Autodesk Inventor part; units mm, degrees
ref_plane "YZ Plane" through (0, 0, 0) normal (1, 0, 0) x (0, 1, 0)
ref_plane "XZ Plane" through (0, 0, 0) normal (0, 1, 0) x (-1, 0, 0)
ref_plane "XY Plane" through (0, 0, 0) normal (0, 0, 1) x (1, 0, 0)
sketch "Skizze1" plane through (0, 0, 0) normal (0, 0, 1) x (1, 0, 0)
  line L0 (-126, 0) -> (126, 0)
  line L1 (0, -126) -> (0, 126)
  line L2 (-90, 4.7809) -> (90, 4.7809)
  line L3 (90, 4.7809) -> (90, -5.2191)
  line L4 (90, -5.2191) -> (-90, -5.2191)
  line L5 (-90, -5.2191) -> (-90, 4.7809)
  line L6 (-4.0898, 90) -> (5.9102, 90)
  line L7 (5.9102, 90) -> (5.9102, -90)
  line L8 (5.9102, -90) -> (-4.0898, -90)
  line L9 (-4.0898, -90) -> (-4.0898, 90)
  point P0 (0, 0)
  point P1 (-4.0898, 4.7809)
  point P2 (-4.0898, -5.2191)
  point P3 (5.9102, -5.2191)
  point P4 (5.9102, 4.7809)
  dimension "d0" = 10
  dimension "d1" = 180
  dimension "d2" = 90
  dimension "d3" = 10
  dimension "d4" = 180
  dimension "d5" = 90
extrude "Extrusion1" add sketch "Skizze1" along normal blind 190
sketch "Skizze2" plane through (0, 0, 0) normal (0, 0, -1) x (-1, 0, 0)
  line L0 (-90, 4.7809) -> (-5.9102, 4.7809)
  line L1 (90, -5.2191) -> (4.0898, -5.2191)
  line L2 (-5.9102, 4.7809) -> (4.0898, 4.7809)
  line L3 (4.0898, 4.7809) -> (4.0898, -5.2191)
  line L4 (4.0898, -5.2191) -> (-5.9102, -5.2191)
  line L5 (-5.9102, -5.2191) -> (-5.9102, 4.7809)
  point P0 (0, 0)
extrude "Extrusion2" add sketch "Skizze2" along normal blind 7
properties part number "Gitter"
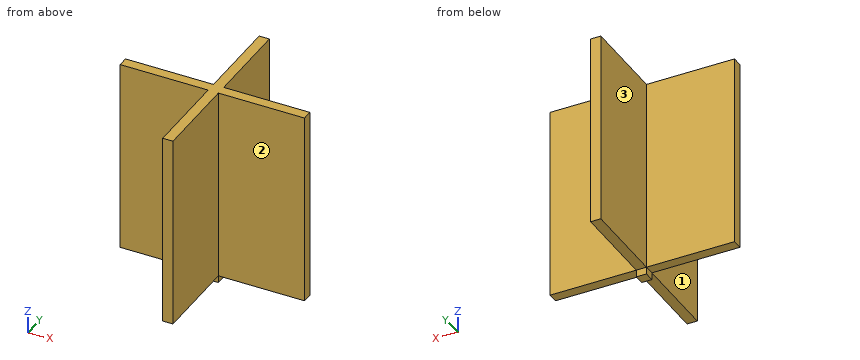
Check sheet for the modelled part. Datum: model origin and axes. Units: mm. Face numbers are marked on the shaded views. A direction names the side the tool comes from. Coordinates: 2 decimals unless noted, no trailing zeros. Write each loop counter-clockwise with the first axis right and the second up, starting at its lowest first coordinate (ties: lowest second). Pieces come first, ordered by that corner, then holes. Notation, with made-up numbers: (-30.75, -22.75) -> (-7.75, -22.75) arc R23 cw to (-7.75, -1.75) -> close; hole circle Ø8 at (54.25, 13.5). An arc over 180 degrees is marked (long way). Use a Markdown table: item, result.
1. Go/stop test with flat-tipped pins: pin 1 Ø10 at (x, z) = (-26, 20.5) entering from -Y; pin 2 Ø3.5 at (y, z) = (0.5, -2) entering from +X; pin 3 Ø3 at (x, y) = (1.5, 57) entering from -Z. Record where each tip stops, or that it passes through.
Reported:
| item | result |
|---|---|
| pin 1 | stops at y = -5.22 |
| pin 2 | stops at x = 5.91 |
| pin 3 | stops at z = 0 |
2. Sectioned sample at C-C (y = 53). Enter the section's corners in (x, z), plus the area to 3 significant figures.
Reported:
| item | result |
|---|---|
| outline | (-4.09, 0) -> (5.91, 0) -> (5.91, 190) -> (-4.09, 190) -> close |
| area | 1,900 mm2 |
3. Scan lines: line 1 along Y through (x, z) = (-68.5, 155.5); line 2 along X through (y, z) = (-51, 109). Record each from-to range of solid material in increasing order.
Reported:
| item | result |
|---|---|
| line 1 | y = -5.22 to 4.78 |
| line 2 | x = -4.09 to 5.91 |
4. Tool access check on the marked faces 1, 2 and 3. Record the directions out of +Z, -Z, +X, -X, +Y, -Y that give a thin tool (end or side, any length) a straight path to the whole face; none if there is none.
Reported:
| item | result |
|---|---|
| face 1 | +Z, -Z, -X, -Y |
| face 2 | +Z, -Z, +X, -Y |
| face 3 | +Z, -Z, -X, +Y |
5. Sectioned sample at A-A (z = 96). Enter the section's corners in (x, y), plus the area to 3 significant figures.
Reported:
| item | result |
|---|---|
| outline | (-90, -5.22) -> (-4.09, -5.22) -> (-4.09, -90) -> (5.91, -90) -> (5.91, -5.22) -> (90, -5.22) -> (90, 4.78) -> (5.91, 4.78) -> (5.91, 90) -> (-4.09, 90) -> (-4.09, 4.78) -> (-90, 4.78) -> close |
| area | 3,500 mm2 |
6. Sectioned sample at B-B (x = 11.5). Enter the section's corners in (y, z).
Reported:
| item | result |
|---|---|
| outline | (-5.22, 0) -> (4.78, 0) -> (4.78, 190) -> (-5.22, 190) -> close |
